Build history of the part. All positions in model axes, mm. A direction names the side the tool comes from. Give positions to 0.01 mm unless a question says otherwise; leave off trailing zeros. Order: outer loops, then holes, each group sorted by start corner. A loop starts at its lowest first (then second) coordinate and runs counter-clockwise, first axis right, second up. Notation, with made-up numbers: (66, -26.75) - (70, -26.75) arc R18 ccw to (70, -2.75) - close; hole circle Ø3 at (54.5, -0.75). An arc over 180 degrees is marked (long way). One line per item, written item: value.
```python
from build123d import *
from build123d.topology import SkipClean

# Parameters (mm, degrees)
SKETCH5_R           = 3
SKETCH5_W           = 236
SKETCH5_H           = 144
BOSS_EXTRUDE1_DEPTH = 10
BOSS_EXTRUDE2_START = 75
SKETCH7_W           = 280.9
SKETCH7_H           = 156
SKETCH7_R           = 3
BOSS_EXTRUDE2_DEPTH = 75
SKETCH9_W           = 5
SKETCH9_H           = 77
SKETCH9_W_2         = 280.9
BOSS_EXTRUDE3_DEPTH = 5
SKETCH10_W          = 5
SKETCH10_H          = 77
BOSS_EXTRUDE5_DEPTH = 120
SKETCH11_R          = 3
CUT_EXTRUDE1_DEPTH  = 1011


with BuildPart() as part:
    # Sketch5 → Boss-Extrude1 (new body)
    with BuildSketch(Plane(origin=(0, 0, 0), x_dir=(1, 0, 0), z_dir=(0, 1, 0))):
        with BuildLine():
            Line((-142.45, 69.9), (-142.45, -71.1))
            ThreePointArc((-142.45, -71.1), (-138.935281374, -79.585281374), (-130.45, -83.1))
            Line((-130.45, -83.1), (130.45, -83.1))
            ThreePointArc((130.45, -83.1), (138.935281374, -79.585281374), (142.45, -71.1))
            Line((142.45, -71.1), (142.45, 69.9))
            ThreePointArc((142.45, 69.9), (138.935281374, 78.385281374), (130.45, 81.9))
            Line((130.45, 81.9), (-130.45, 81.9))
            ThreePointArc((-130.45, 81.9), (-138.935281374, 78.385281374), (-142.45, 69.9))
        make_face()
        with Locations(Location((-122.45, 59.6, 0), (0, 0, 270))):
            Circle(SKETCH5_R, mode=Mode.SUBTRACT)
        with Locations(Location((-122.45, -60.8, 0), (0, 0, 270))):
            Circle(SKETCH5_R, mode=Mode.SUBTRACT)
        with Locations(Location((122.45, -60.8, 0), (0, 0, 270))):
            Circle(SKETCH5_R, mode=Mode.SUBTRACT)
        with Locations(Location((122.45, 59.6, 0), (0, 0, 270))):
            Circle(SKETCH5_R, mode=Mode.SUBTRACT)
        with Locations(Location((-132.45, -0.6, 0), (0, 0, 270))):
            Circle(SKETCH5_R, mode=Mode.SUBTRACT)
        with Locations(Location((132.45, -0.6, 0), (0, 0, 90))):
            Circle(SKETCH5_R, mode=Mode.SUBTRACT)
        Rectangle(SKETCH5_W, SKETCH5_H, mode=Mode.SUBTRACT)
    extrude(amount=BOSS_EXTRUDE1_DEPTH)

    # Sketch7 → Boss-Extrude2 (add)
    with SkipClean():  # the faces are left unmerged after this step: merging them gives an invalid solid
        with BuildSketch(Plane.XZ.offset(BOSS_EXTRUDE2_START)):
            with Locations((0, 0.6)):
                Rectangle(SKETCH7_W, SKETCH7_H)
            with Locations(Location((132.45, 0.6, 0), (0, 0, 270))):
                Circle(SKETCH7_R, mode=Mode.SUBTRACT)
            with Locations(Location((-132.45, 0.6, 0), (0, 0, 270))):
                Circle(SKETCH7_R, mode=Mode.SUBTRACT)
        extrude(amount=-BOSS_EXTRUDE2_DEPTH)



with BuildPart() as body_2:
    # Sketch9 → Boss-Extrude3 (new body)
    with BuildSketch(Plane(origin=(0, -145, 0), x_dir=(-1, 0, 0), z_dir=(0, -1, 0))):
        with Locations((-142.95, 0)):
            Rectangle(SKETCH9_W, SKETCH9_H)
        Rectangle(SKETCH9_W_2, SKETCH9_H)
        with Locations((142.95, 0)):
            Rectangle(SKETCH9_W, SKETCH9_H)
    extrude(amount=BOSS_EXTRUDE3_DEPTH)


with BuildPart() as part_1:
    with SkipClean():  # the faces are left unmerged after this step: merging them gives an invalid solid
        add(part.part)

        add(body_2.part)  # Boss-Extrude5 merges body 2
        # Sketch10 → Boss-Extrude5 (add)
        with BuildSketch(Plane(origin=(0, -145, 0), x_dir=(1, 0, 0), z_dir=(0, 1, 0))):
            with Locations((-142.95, 0)):
                Rectangle(SKETCH10_W, SKETCH10_H)
            with Locations((142.95, 0)):
                Rectangle(SKETCH10_W, SKETCH10_H)
        extrude(amount=BOSS_EXTRUDE5_DEPTH)

    # Sketch11 → Cut-Extrude1 (cut)
    with SkipClean():  # the faces are left unmerged after this step: merging them gives an invalid solid
        with BuildSketch(Plane.ZY.offset(145.45)):
            with Locations((0.3, -37.5)):
                Circle(SKETCH11_R)
        extrude(amount=-CUT_EXTRUDE1_DEPTH, mode=Mode.SUBTRACT)


solid = part_1.part
```
(1) Slice it at C-C, the plane z = 51.5. Give the cut face in (x, y), and give its area (3 significant figures).
Completed:
outline: (-142.45, 0) - (-140.45, 0) - (-140.45, -75) - (140.45, -75) - (140.45, 0) - (142.45, 0) - (142.45, 10) - (118, 10) - (118, 0) - (-118, 0) - (-118, 10) - (-142.45, 10) - close
area: 21,600 mm²
(2) Pin check, flat tips, straight feed: P1, Ø5, axis at x = -107, z = -50, coming from the +Y side; P2, Ø3.5, axis at x = 132.45, z = 0.6, coming from the +Y side; P3, Ø1.5, axis at x = 143.5, z = -5.5, coming from the +Y side. Stop position of each tip, or through.
Completed:
P1: y = 0
P2: y = -145
P3: y = -25
(3) Pull direction X, two halves, no side cores. Call faces 1 (the face through (-119.92, 4.93, 62.41)), 2 (the face through (138.84, 4.93, 79.68)), 3 (the face through (-2, -37.4, -2.7)): +X half, -X half, draft (parallel to the pull), parting line (faces both ways), or undercut.
Completed:
face 1: undercut
face 2: +X half
face 3: draft
(4) Drill centre lines: line 1 (Y direction, x = -43.5, z = 0.3); line 2 (X direction, y = 3.75, z = 60.8); line 3 (X direction, y = 4, z = 60). Where is each one in solid material? Low to high.
Completed:
line 1: -150 to -145, -75 to -40.5, -34.5 to 0
line 2: -142.45 to -125.45, -119.45 to -118, 118 to 119.45, 125.45 to 142.45
line 3: -142.45 to -125.34, -119.56 to -118, 118 to 119.56, 125.34 to 142.45
(5) 3-axis set-ups, long thin cutter, end or side, ignore diameter. For faces 4 (the face through (-142.45, 5, 0)), 5 (the face through (-2, -38, -77.4)), 6 (the face through (-2, 0, 1)): which of +Z, -Z, +X, -X, +Y, -Y reach the whole face in a straight line?
Completed:
face 4: +Z, -Z, -X, +Y
face 5: -Z, +X, -X, -Y
face 6: +Y
(6) Slice it at B-B, the plane y = -127. Give the cut face in (x, z).
Completed:
outline: (-145.45, -38.5) - (-140.45, -38.5) - (-140.45, 38.5) - (-145.45, 38.5) - close; (140.45, -38.5) - (145.45, -38.5) - (145.45, 38.5) - (140.45, 38.5) - close
(7) Slice it at A-A, the plane x = -5. Give the cut face in (y, z), and give its area (3 significant figures).
Completed:
outline: (-150, -38.5) - (-145, -38.5) - (-145, 38.5) - (-150, 38.5) - close; (-75, -77.4) - (0, -77.4) - (0, -81.9) - (10, -81.9) - (10, -72) - (0, -72) - (0, 72) - (10, 72) - (10, 83.1) - (0, 83.1) - (0, 78.6) - (-75, 78.6) - close; hole circle Ø6 at (-37.5, 0.3)
area: 12,300 mm²
(8) Slice it at D-D, the plane y = -65. Give the cut face in (x, z), and give its area (3 significant figures).
Completed:
outline: (-145.45, -38.5) - (-140.45, -38.5) - (-140.45, -77.4) - (140.45, -77.4) - (140.45, -38.5) - (145.45, -38.5) - (145.45, 38.5) - (140.45, 38.5) - (140.45, 78.6) - (-140.45, 78.6) - (-140.45, 38.5) - (-145.45, 38.5) - close; hole circle Ø6 at (-132.45, 0.6); hole circle Ø6 at (132.45, 0.6)
area: 44,500 mm²
